Can you work these out from the drawing? Everything is in mm from the part's minimum corner. Give positions to 0.01 mm unless a question says otherwise; leave off trailing zeros. Write each loop counter-clockwise with the first axis right and the second up, starting at its lowest first coordinate (ties: lowest second). Pieces come first, ordered by that corner, then holes. Notation, with made-up numbers: (-15, -28.75) -> (11, -28.75) arc R28 cw to (11, 3.25) -> close; hole circle Ø5 at (8, 17.25). An arc over 180 degrees is marked (long way). Use one line per item in the form item = value.
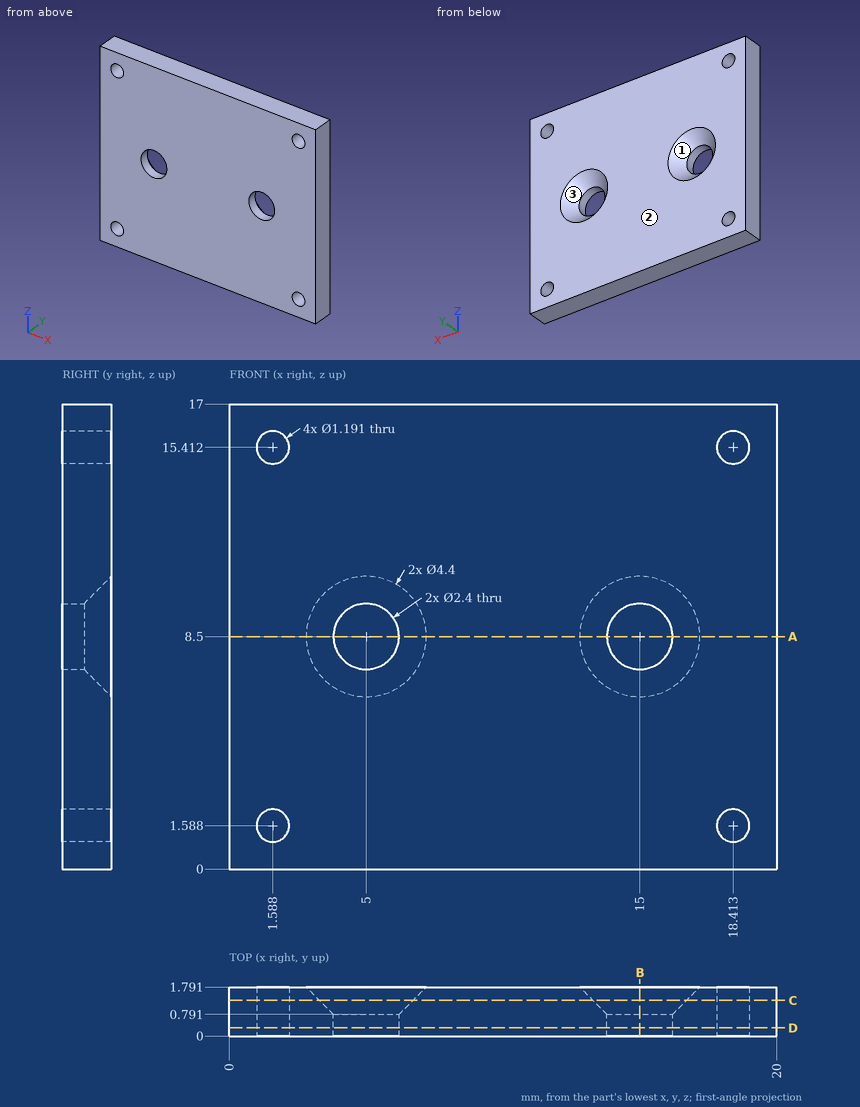
Q1. I want a section at A-A, the plane z = 8.5. Write out the boundary of the cut face in (x, y).
Result set:
outline = (0, 0) -> (3.8, 0) -> (3.8, 0.79) -> (2.8, 1.79) -> (0, 1.79) -> close; (6.2, 0) -> (13.8, 0) -> (13.8, 0.79) -> (12.8, 1.79) -> (7.2, 1.79) -> (6.2, 0.79) -> close; (16.2, 0) -> (20, 0) -> (20, 1.79) -> (17.2, 1.79) -> (16.2, 0.79) -> close
Q2. I want a section at B-B, the plane x = 15. Write out the boundary of the cut face in (y, z).
Result set:
outline = (0, 0) -> (1.79, 0) -> (1.79, 6.3) -> (0.79, 7.3) -> (0, 7.3) -> close; (0, 9.7) -> (0.79, 9.7) -> (1.79, 10.7) -> (1.79, 17) -> (0, 17) -> close
Q3. I want a section at C-C, the plane y = 1.3. Write out the boundary of the cut face in (x, z) (1 decimal), and give its area (3 significant figures).
Result set:
outline = (0, 0) -> (20, 0) -> (20, 17) -> (0, 17) -> close; hole circle Ø1.2 at (1.6, 1.6); hole circle Ø1.2 at (1.6, 15.4); hole circle Ø3.4 at (5, 8.5); hole circle Ø3.4 at (15, 8.5); hole circle Ø1.2 at (18.4, 1.6); hole circle Ø1.2 at (18.4, 15.4)
area = 317 mm2
Q4. If we mould it in two halves opening along X, with no side actions, what happens to the marked faces 1, 2 and 3? For each: +X half, -X half, draft (parallel to the pull), parting line (faces both ways), or undercut.
Result set:
face_1 = undercut
face_2 = draft
face_3 = undercut
Q5. I want a section at D-D, the plane y = 0.3. Write out the boundary of the cut face in (x, z) (1 decimal).
Result set:
outline = (0, 0) -> (20, 0) -> (20, 17) -> (0, 17) -> close; hole circle Ø1.2 at (1.6, 1.6); hole circle Ø1.2 at (1.6, 15.4); hole circle Ø2.4 at (5, 8.5); hole circle Ø2.4 at (15, 8.5); hole circle Ø1.2 at (18.4, 1.6); hole circle Ø1.2 at (18.4, 15.4)
Q6. Will this pin go through, and if not, where does the flat tip stop? pin 1 Ø1.9 at (x, z) = (15, 8.5) entering from -Y.
Result set:
pin_1 = through
Q7. If I drill on line 1 along X through (y, z) = (0.45, 8.5); line 2 along Z through (x, y) = (15, 0.2); line 3 along X through (y, z) = (0.7, 9.5) (1 decimal), over which ranges is the centre line in solid material (lowest first)? Write a range as from..to.
Result set:
line_1 = 0..3.8, 6.2..13.8, 16.2..20
line_2 = 0..7.3, 9.7..17
line_3 = 0..4.3, 5.7..14.3, 15.7..20
